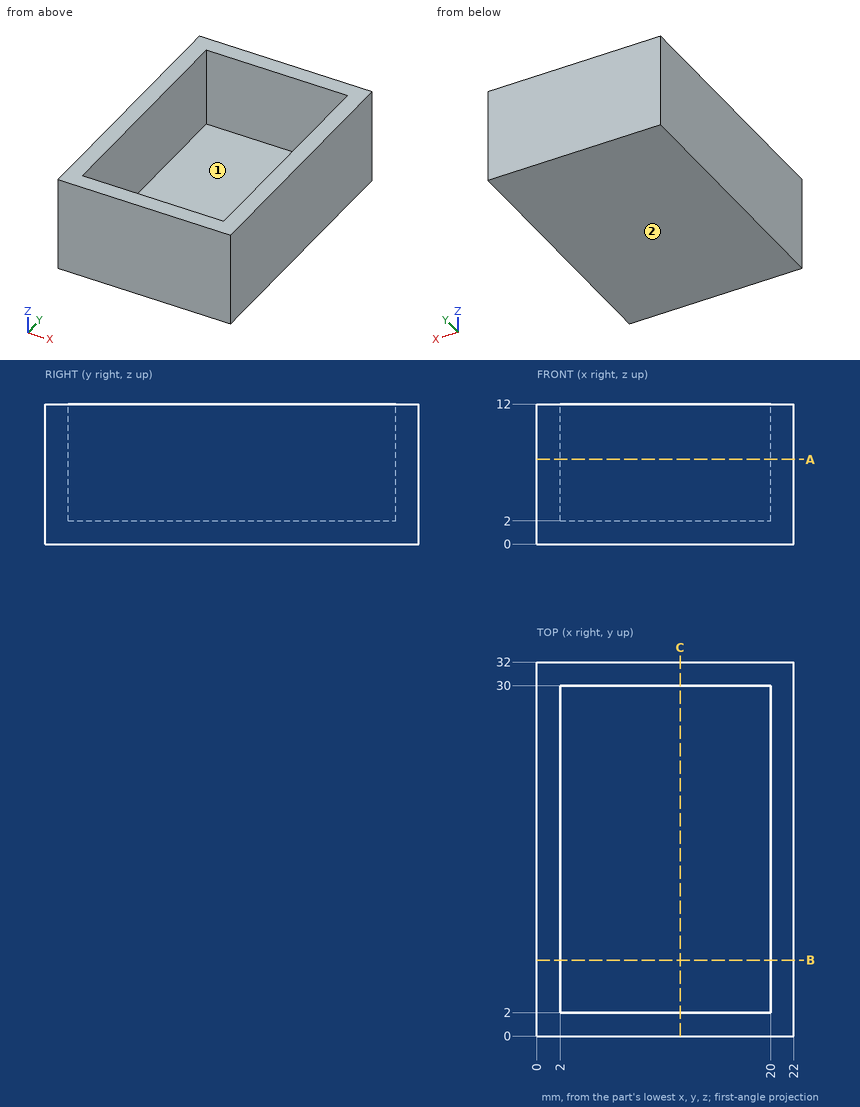
Verification items for this drawing (mm, ordinates from the low corner). A direction names the side the tool comes from. Round coordinates to 2 decimals unless told otherwise and drop trailing zeros. Loops run counter-clockwise (first coordinate to the right, second up) from the corner with the lowest first, then second, coordinate; pieces in that order, holes last. Notation, with made-up numbers: (-13, 50) -> (8, 50) arc R8 cw to (8, 61) -> close; hole circle Ø4 at (71, 51). An arc over 180 degrees is marked (long way). Answer in a Markdown table with one row per item.
Q1. Set-up check for the marked faces 1 and 2: record each of +Z, -Z, +X, -X, +Y, -Y from which the full face is reachable in a straight line by a thin tool's end or side.
Data:
| item | result |
|---|---|
| face 1 | +Z |
| face 2 | -Z, +X, -X, +Y, -Y |
Q2. Go/stop test with a flat-tipped pin: P1, Ø12, axis at x = 11.5, y = 16, coming from the +Z side. Record where the tip stops, or that it passes through.
Data:
| item | result |
|---|---|
| P1 | stops at z = 2 |
Q3. Sectioned sample at B-B on y = 6.5. Enter the section's corners in (x, z), then the cut area to 3 significant figures.
Data:
| item | result |
|---|---|
| outline | (0, 0) -> (22, 0) -> (22, 12) -> (20, 12) -> (20, 2) -> (2, 2) -> (2, 12) -> (0, 12) -> close |
| area | 84.0 mm^2 |
Q4. Sectioned sample at C-C on x = 12.25. Enter the section's corners in (y, z), then the cut area to 3 significant figures.
Data:
| item | result |
|---|---|
| outline | (0, 0) -> (32, 0) -> (32, 12) -> (30, 12) -> (30, 2) -> (2, 2) -> (2, 12) -> (0, 12) -> close |
| area | 104 mm^2 |
Q5. Sectioned sample at A-A on z = 7.25. Enter the section's corners in (x, y).
Data:
| item | result |
|---|---|
| outline | (0, 0) -> (22, 0) -> (22, 32) -> (0, 32) -> close; hole (2, 2) -> (20, 2) -> (20, 30) -> (2, 30) -> close |
Q6. Thickness scan on L1, parallel to X at y = 28, z = 2.5; L2, parallel to Y at x = 8.25, z = 11; L3, parallel to Z at x = 7, y = 13.5. Record the ranges inside material, lowest first.
Data:
| item | result |
|---|---|
| L1 | x = 0 to 2, 20 to 22 |
| L2 | y = 0 to 2, 30 to 32 |
| L3 | z = 0 to 2 |
